Input: dimensioned drawing with shaded views. Units: mm. Origin: part minimum x, y, z. Round coordinates to 2 decimals unless told otherwise and drop trailing zeros. Loops run counter-clockwise (first coordinate to the right, second up) from the corner with the lowest first, then second, coordinate; pieces in that order, holes last. Notation, with made-up numbers: M -17.5,-18.75 L 14.5,-18.75 A30 cw 14.5,8.25 Z; hole C 59,-19 d1. An arc over 180 degrees is marked long. Answer as a JSON object with one key per item and string values.
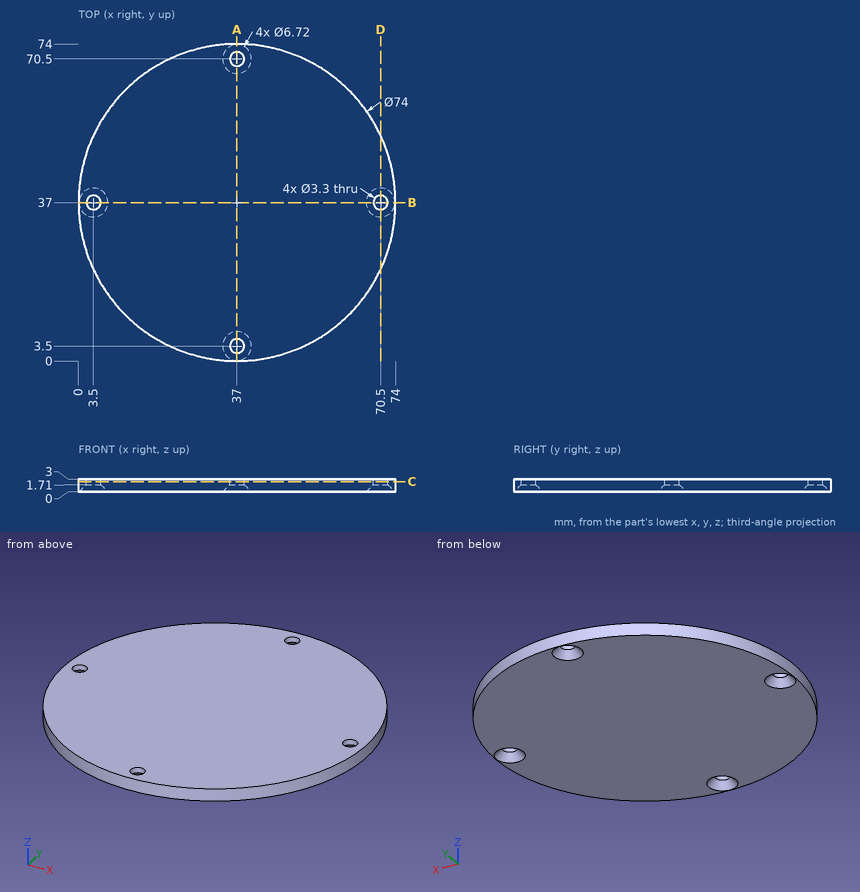
Item 1: Line query: probe 1 along Y at (x, z) = (37, 2.2); probe 2 along X at (y, z) = (36, 0.15); probe 3 along Y at (x, z) = (3.5, 2). Output: solid intervals per line, ascending. Write a range as from..to.
Answer sheet:
{"probe 1": "y = 0..1.85, 5.15..68.85, 72.15..74", "probe 2": "x = 0.01..0.45, 6.55..67.45, 73.55..73.99", "probe 3": "y = 21.29..35.35, 38.65..52.71"}
Item 2: Section C-C on z = 2.4. Return the cut outline in (x, y).
Answer sheet:
{"outline": "C 37,37 d74; hole C 3.5,37 d3.3; hole C 37,3.5 d3.3; hole C 37,70.5 d3.3; hole C 70.5,37 d3.3"}
Item 3: Contact query for flat-ended pins moving along their axis: pin 1 Ø1.5 at (y, z) = (20.5, 1) entering from -X; pin 2 Ø2.5 at (x, y) = (37, 3.5) entering from +Z; pin 3 Ø1.5 at (x, z) = (38.5, 1) entering from +Y; pin 4 Ø1 at (y, z) = (66.5, 1) entering from -X. Output: stop coordinate, or through.
Answer sheet:
{"pin 1": "stops at x = 3.52", "pin 2": "passes through", "pin 3": "stops at y = 73.99", "pin 4": "stops at x = 14.02"}
Item 4: Section D-D on x = 70.5. Return the cut outline in (y, z), then the cut area to 3 significant figures.
Answer sheet:
{"outline": "M 21.29,0 L 33.64,0 L 35.35,1.71 L 35.35,3 L 21.29,3 Z; M 38.65,1.71 L 40.36,0 L 52.71,0 L 52.71,3 L 38.65,3 Z", "area": "81.4 mm²"}
Item 5: Section A-A on x = 37. Return the cut outline in (y, z), then the cut area to 3 significant figures.
Answer sheet:
{"outline": "M 0,0 L 0.14,0 L 1.85,1.71 L 1.85,3 L 0,3 Z; M 5.15,1.71 L 6.86,0 L 67.14,0 L 68.85,1.71 L 68.85,3 L 5.15,3 Z; M 72.15,1.71 L 73.86,0 L 74,0 L 74,3 L 72.15,3 Z", "area": "196 mm²"}
